from build123d import *

# Parameters (mm, degrees)
BOSS_EXTRUDE1_DEPTH = 17.78
SKETCH2_W           = 41
SKETCH2_H           = 20.4
CUT_EXTRUDE1_DEPTH  = 1.27
SKETCH3_W           = 7.62
SKETCH3_H           = 12.7
CUT_EXTRUDE2_DEPTH  = 2.54
SKETCH4_W           = 50.8
SKETCH4_H           = 20.32
SKETCH4_W_2         = 20.32
SKETCH4_H_2         = 50.8
CUT_EXTRUDE3_DEPTH  = 2.54


with BuildPart() as part:
    # Sketch1 → Boss-Extrude1 (new body)
    with BuildSketch(Plane(origin=(0, 0, 0), x_dir=(1, 0, 0), z_dir=(0, 1, 0))):
        with BuildLine():
            Line((50.8, -42.084097937), (-50.8, -42.084097937))
            Line((-50.8, -42.084097937), (-50.8, -143.684097937))
            ThreePointArc((-50.8, -143.684097937), (-135.481402596, -69.789322613), (-146.480963287, 42.060520616))
            Line((-146.480963287, 42.060520616), (-50.866637556, 42.060520616))
            Line((-50.866637556, 42.060520616), (-50.866637556, 143.660520616))
            ThreePointArc((-50.866637556, 143.660520616), (-0.035342799, 152.399995902), (50.8, 143.684097937))
            Line((50.8, 143.684097937), (50.8, 42.060520616))
            Line((50.8, 42.060520616), (146.480963287, 42.060520616))
            ThreePointArc((146.480963287, 42.060520616), (135.481402596, -69.789322613), (50.8, -143.684097937))
            Line((50.8, -143.684097937), (50.8, -42.084097937))
        make_face()
    extrude(amount=BOSS_EXTRUDE1_DEPTH)

    # Sketch2 → Cut-Extrude1 (cut)
    with BuildSketch(Plane(origin=(0, 17.78, 0), x_dir=(1, 0, 0), z_dir=(0, 1, 0))):
        with Locations((0, 31.598605784)):
            Rectangle(SKETCH2_W, SKETCH2_H)
    extrude(amount=-CUT_EXTRUDE1_DEPTH, mode=Mode.SUBTRACT)

    # Sketch3 → Cut-Extrude2 (cut)
    with BuildSketch(Plane(origin=(0, 17.78, 0), x_dir=(1, 0, 0), z_dir=(0, 1, 0))):
        with Locations((-62.23, -80.184097937)):
            Rectangle(SKETCH3_W, SKETCH3_H)
        with Locations((62.23, -80.184097937)):
            Rectangle(SKETCH3_W, SKETCH3_H)
    extrude(amount=-CUT_EXTRUDE2_DEPTH, mode=Mode.SUBTRACT)

    # Sketch4 → Cut-Extrude3 (cut)
    with BuildSketch(Plane(origin=(0, 17.78, 0), x_dir=(1, 0, 0), z_dir=(0, 1, 0))):
        with Locations((-98.673800421, 28.511480762)):
            Rectangle(SKETCH4_W, SKETCH4_H)
        with Locations((98.673800421, 28.511480762)):
            Rectangle(SKETCH4_W, SKETCH4_H)
        with Locations((-40.485390627, -10.503849142)):
            Rectangle(SKETCH4_W_2, SKETCH4_H_2)
        with Locations((40.485644605, -10.503849142)):
            Rectangle(SKETCH4_W_2, SKETCH4_H_2)
    extrude(amount=-CUT_EXTRUDE3_DEPTH, mode=Mode.SUBTRACT)


solid = part.part
Source: CAD feature listing. Evaluate the final solid. Frame: model axes, mm. A direction names the side the tool comes from. Give positions to 0.01 mm unless a question says otherwise; leave off trailing zeros. Write each loop counter-clockwise with the first axis right and the second up, starting at its lowest first coordinate (ties: lowest second). Pieces come first, ordered by that corner, then holes. Notation, with made-up numbers: M 24.5,37.5 L 54.5,37.5 A12 cw 54.5,55.5 Z; hole C 51.5,23 d2. An arc over 180 degrees is marked long. Return JSON: item names as keys, results as strings. Group by question number.
1) Cut plane B-B, the plane y = 8.25. Output: boundary loops of the cut face in (x, z).
2) Cut plane C-C, the plane x = -108.5. Output: boundary loops of the cut face in (y, z).
3) Cut plane A-A, the plane z = 109.5. Output: boundary loops of the cut face in (x, y), plus the area to 3 significant figures.
4) Material intervals for line 1 along X through (y, z) = (13.25, -71.5); line 2 along Z through (x, y) = (-109.5, 17); line 3 along Y through (x, z) = (100.5, -36), sorted ascending. Write a range as [from, to].
5) Cut plane D-D, the plane z = 32.5. Output: boundary loops of the cut face in (x, y).
6) Pull-direction query (X, two-part tool) for faces 5 (the face through (50.8, 9, 94)), 6 (the face through (-50.867, 9, -92)), 7 (the face through (-0.76, 8.77, -152.4)), 8 (the face through (50.8, 9, -94)); classes: pulls with the +X half, pulls with the -X half, needs draft (parallel to the pull), parting line crosses it, or undercut.
7) Pin query (flat end, axial travel): P1, Ø2, axis at x = -45, y = 16.5, coming from the +Z side; P2, Ø10, axis at x = -44.5, z = 51, coming from the +Y side; P3, Ø3, axis at y = 16.5, z = -29.5, coming from the +X side; P4, Ø0.8, axis at x = -86, y = 16.5, coming from the +Z side. Return the tip coordinate at first contact, or that it passes through.
8) Set-up query: faces 1 (the face through (1, 9, 42.084)), 2 (the face through (-99, 9, -42.061)), 3 (the face through (62, 15.24, 80)), 4 (the face through (98, 9, -42.061)). Return all of +Z, -Z, +X, -X, +Y, -Y with unobstructed straight access to the full face (end or side cutting, diameter ignored); none if empty.
Recorded:
{
 "1": {"outline": "M -146.48,-42.06 L -50.87,-42.06 L -50.87,-143.66 A152.4 ccw 50.8,-143.68 L 50.8,-42.06 L 146.48,-42.06 A152.4 ccw 50.8,143.68 L 50.8,42.08 L -50.8,42.08 L -50.8,143.68 A152.4 ccw Z"},
 "2": {"outline": "M 0,-42.06 L 17.78,-42.06 L 17.78,-38.67 L 15.24,-38.67 L 15.24,-18.35 L 17.78,-18.35 L 17.78,107.02 L 0,107.02 Z"},
 "3": {"outline": "M -106,0 L -50.8,0 L -50.8,17.78 L -106,17.78 Z; M 50.8,0 L 106,0 L 106,17.78 L 50.8,17.78 Z", "area": "1,960 mm²"},
 "4": {"line 1": "x = [-50.87, 50.8]", "line 2": "z = [-42.06, -38.67], [-18.35, 106]", "line 3": "y = [0, 15.24]"},
 "5": {"outline": "M -148.89,0 L 148.89,0 L 148.89,17.78 L 50.65,17.78 L 50.65,15.24 L 30.33,15.24 L 30.33,17.78 L -30.33,17.78 L -30.33,15.24 L -50.65,15.24 L -50.65,17.78 L -148.89,17.78 Z"},
 "6": {"face 5": "undercut", "face 6": "pulls with the -X half", "face 7": "parting line crosses it", "face 8": "pulls with the +X half"},
 "7": {"P1": "stops at z = 42.08", "P2": "passes through", "P3": "stops at x = 149.81", "P4": "stops at z = 126.09"},
 "8": {"face 1": "+Z, +Y, -Y", "face 2": "-Z, -X, +Y, -Y", "face 3": "+Y", "face 4": "-Z, +X, +Y, -Y"}
}
